Check sheet for the drawn part. Datum: minimum x, y, z corner. Units: mm. Give positions to 0.01 mm unless a question says otherwise; leave off trailing zeros. Order: outer loops, then holes, each group sorted by start corner. A loop starts at its lowest first (then second) coordinate and runs counter-clockwise, first axis right, second up. Notation, with made-up numbers: (34, 56.25) -> (66, 56.25) arc R16 cw to (66, 78.25) -> close; hole circle Ø1 at (-5.75, 43.25). An arc over 180 degrees is marked (long way). Answer in a Markdown table with one row per item. Add a question column.
(1) Cross-section at B-B (x = 116). Record the cut outline in (y, z).
(2) Cross-section at A-A (z = 6.5). Record the cut outline in (x, y).
(3) Thickness scan on L1, parallel to X at y = 4.75, z = 6; L2, parallel to Z at x = 84.5, y = 2; L3, parallel to Y at x = 30, z = 3.3. Record the ranges inside material, lowest first. Write a range as [from, to].
(4) Go/stop test with flat-tipped pins: pin 1 (2 mm diameter, centred on x = 30, y = 6, fed in from +Z); pin 2 (1 mm diameter, centred on x = 90, y = 6, fed in from +Z). Record where each tip stops, or that it passes through.
(5) Release check for a two-part mould opening along X. For the marked faces 1, 2 and 3 record: released by +X, released by -X, zero draft, split by the parting line, or undercut.
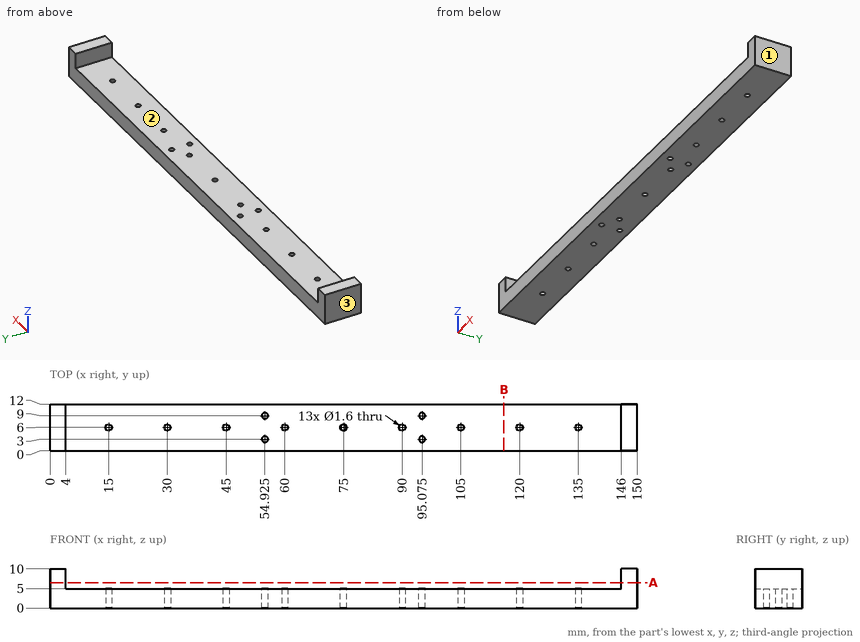
Answer below:
| question | item | result |
|---|---|---|
| 1 | outline | (0, 0) -> (12, 0) -> (12, 5) -> (0, 5) -> close |
| 2 | outline | (0, 0) -> (4, 0) -> (4, 12) -> (0, 12) -> close; (146, 0) -> (150, 0) -> (150, 12) -> (146, 12) -> close |
| 3 | L1 | x = [0, 4], [146, 150] |
| 3 | L2 | z = [0, 5] |
| 3 | L3 | y = [0, 5.2], [6.8, 12] |
| 4 | pin 1 | stops at z = 5 |
| 4 | pin 2 | passes through |
| 5 | face 1 | released by +X |
| 5 | face 2 | undercut |
| 5 | face 3 | released by -X |
